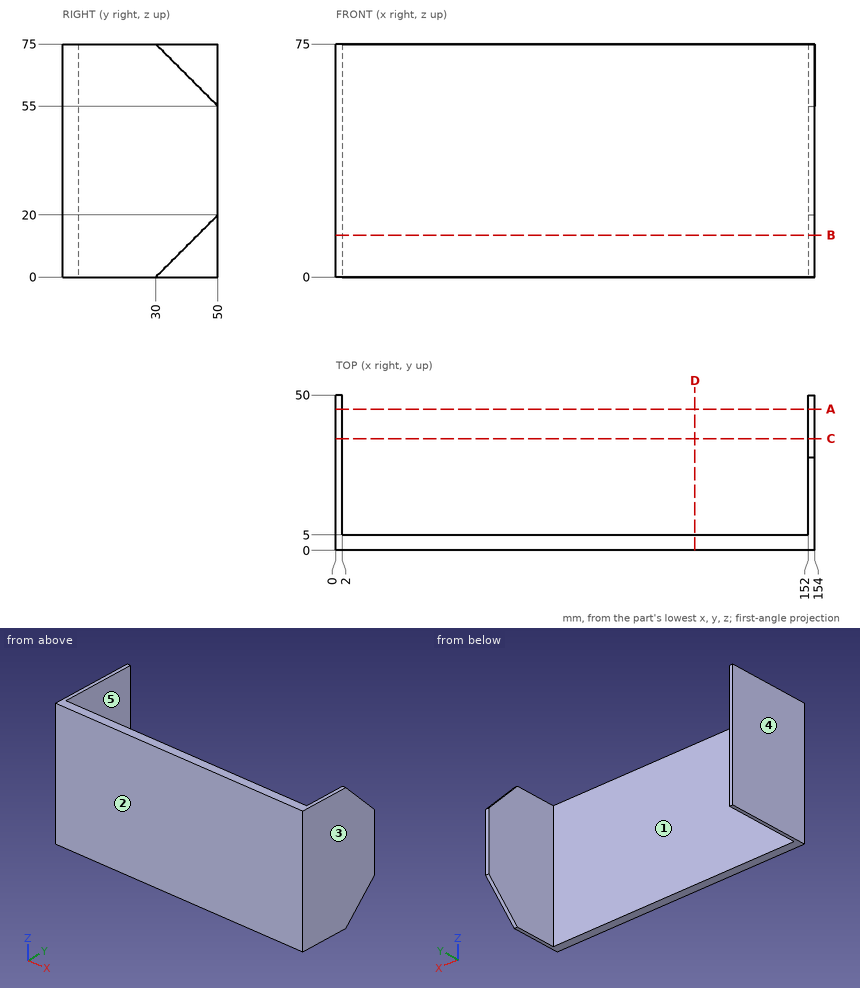
Study the drawing (mm; zero at the part's minimum x, y, z) and answer. A direction names the side the tool comes from. Give positions to 0.01 mm unless a question says otherwise; leave off trailing zeros. Write each loop counter-clockwise with the first axis right and the second up, starting at its lowest first coordinate (ties: lowest second). Pieces come first, ordered by that corner, then holes.
(1) The part is cut by section D-D on x = 115.5. Write down the section's boundary in (y, z).
Final values:
outline: (0, 0) - (5, 0) - (5, 75) - (0, 75) - close
(2) The part is cut by section C-C on y = 36. Write down the section's boundary in (x, z), plus the area to 3 significant figures.
Final values:
outline: (0, 0) - (2, 0) - (2, 75) - (0, 75) - close; (152, 6) - (154, 6) - (154, 69) - (152, 69) - close
area: 276 mm2
(3) The mould has two halves that part along X. Classify the marked faces 3, 4 and 5: pulls with the +X half, pulls with the -X half, needs draft (parallel to the pull), parting line crosses it, or undercut.
Final values:
face 3: pulls with the +X half
face 4: pulls with the -X half
face 5: undercut
(4) Straight lines are drawn through the part: line 1 (X direction, y = 23, z = 60); line 2 (Y direction, x = 43, z = 10). For each, find the intervals that lie inside material, in ascending order.
Final values:
line 1: x = 0 to 2, 152 to 154
line 2: y = 0 to 5
(5) Which of the six approach directions +Z, -Z, +X, -X, +Y, -Y give full straight-line access (tool end or side, diameter ignored) to the marked faces 1 and 2?
Final values:
face 1: +Z, -Z, +Y
face 2: +Z, -Z, +X, -X, -Y
(6) A flat-ended cylindrical pin translates along its axis: pin 1 Ø4 at (x, z) = (112, 57.5) entering from +Y. Find the tip coordinate at first contact, or state that the pin passes through.
Final values:
pin 1: stops at y = 5
(7) The part is cut by section A-A on y = 45.5. Write down the section's boundary in (x, z).
Final values:
outline: (0, 0) - (2, 0) - (2, 75) - (0, 75) - close; (152, 15.5) - (154, 15.5) - (154, 59.5) - (152, 59.5) - close
(8) The part is cut by section B-B on z = 13.5. Write down the section's boundary in (x, y).
Final values:
outline: (0, 0) - (154, 0) - (154, 43.5) - (152, 43.5) - (152, 5) - (2, 5) - (2, 50) - (0, 50) - close
